Design review of the part built by this model. Coordinates are the model's own, in mm. Face numbers are marked on the shaded views. A direction names the side the tool comes from. Coordinates: 2 decimals unless noted, no trailing zeros. Order: outer loops, then holes, each group sorted by start corner. A loop starts at its lowest first (then second) coordinate and runs counter-clockwise, first axis right, second up. Notation, with made-up numbers: (-3.75, -17) -> (43.25, -17) arc R15 ccw to (43.25, 11) -> close; hole circle Ø11 at (18.5, -10.75). An arc over 180 degrees is marked (long way). Write item = value, one per line.
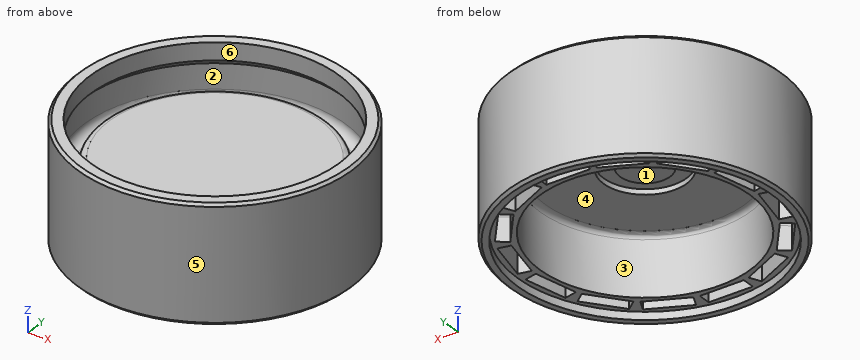
```python
from build123d import *

# Parameters (mm, degrees)
F0_R            = 26
F1_DEPTH        = 22
F2_W            = 8.4
F2_H            = 2.4
F3_DEPTH        = 10
F3_COPIES_COUNT = 14
F4_R            = 4
F5_R            = 20
F6_DEPTH        = 13
F7_R            = 7.9
F8_DEPTH        = 1
F9_R            = 4.75
F10_DEPTH       = 0.8
F11_R           = 23.6
F12_DEPTH       = 7
F13_R           = 24.8
F13_R_2         = 21.2
F14_DEPTH       = 4
F14_DEPTH_BACK  = 4
F15_R           = 1.79999
F16_R           = 1.2
F17_S5_R        = 23.6
F17_T6_DEPTH    = 37
F18_R           = 1
F19_SIZE        = 0.5
F20_R           = 24.3
F21_DEPTH       = 1.5


# Not quite as in the source:
# - a fillet or chamfer that OpenCascade refuses, or shapes differently, is made with other operations: its cross-section is extruded or revolved along the edge and cut away or added
# - a fillet or chamfer is up to 0.001 mm smaller than in the source, because OpenCascade refuses the exact size
# - a pattern or mirror of a feature is missing from the dataset's text; its kind, count and spacing are read off the source's solid


with BuildPart() as f1:
    # F0 (on Top) → F1 (new body)
    with BuildSketch(Plane.XY):
        Circle(F0_R)
    extrude(amount=F1_DEPTH)

    # F2 (on face) → F3 (cut)
    with BuildSketch(Plane(origin=(0, 0, 0), x_dir=(1, 0, 0), z_dir=(0, 0, -1))):
        with Locations((0, 22)):
            Rectangle(F2_W, F2_H)
    f3 = extrude(amount=-F3_DEPTH, mode=Mode.SUBTRACT)

    # F3_copies: F3 ×14 about axis
    f3_copies_axis = Axis((0, 0, 0), (0, 0, 1))
    for i in range(1, F3_COPIES_COUNT):
        add(f3.rotate(f3_copies_axis, i * 360 / F3_COPIES_COUNT), mode=Mode.SUBTRACT)

    # F4
    f4_edges = [f1.edges().sort_by_distance(p)[0] for p in [
        (4.2, -22, 10),
        (-4.2, -22, 10),
        (-19.81895, -10.433083, 10),
        (-14.581635, -17.000468, 10),
        (-13.329512, -17.999003, 10),
        (-5.761373, -21.643627, 10),
        (-22.383002, -0.800763, 10),
        (-20.513826, -8.990158, 10),
        (5.761373, -21.643627, 10),
        (13.329512, -17.999003, 10),
        (14.581635, -17.000468, 10),
        (19.81895, -10.433083, 10),
        (20.513826, -8.990158, 10),
        (22.383002, -0.800763, 10),
        (-20.513826, 8.990158, 10),
        (-22.383002, 0.800763, 10),
        (-14.581635, 17.000468, 10),
        (-19.81895, 10.433083, 10),
        (-5.761373, 21.643627, 10),
        (-13.329512, 17.999003, 10),
        (22.383002, 0.800763, 10),
        (20.513826, 8.990158, 10),
        (4.2, 22, 10),
        (-4.2, 22, 10),
        (13.329512, 17.999003, 10),
        (5.761373, 21.643627, 10),
        (19.81895, 10.433083, 10),
        (14.581635, 17.000468, 10),
    ]]
    fillet(f4_edges, radius=F4_R)

    # F5 (on face) → F6 (cut)
    with BuildSketch(Plane(origin=(0, 0, 0), x_dir=(1, 0, 0), z_dir=(0, 0, -1))):
        Circle(F5_R)
    extrude(amount=-F6_DEPTH, mode=Mode.SUBTRACT)

    # F7 (on face) → F8 (cut)
    with BuildSketch(Plane(origin=(0, 0, 13), x_dir=(1, 0, 0), z_dir=(0, 0, -1))):
        Circle(F7_R)
    extrude(amount=-F8_DEPTH, mode=Mode.SUBTRACT)

    # F9 (on face) → F10 (join)
    with BuildSketch(Plane(origin=(0, 0, 14), x_dir=(1, 0, 0), z_dir=(0, 0, -1))):
        Circle(F9_R)
    extrude(amount=F10_DEPTH)

    # F11 (on face) → F12 (cut)
    with BuildSketch(Plane.XY.offset(22)):
        Circle(F11_R)
    extrude(amount=-F12_DEPTH, mode=Mode.SUBTRACT)

    # F13 (on face) → F14 (cut, two sides)
    with BuildSketch(Plane.XY.offset(15)) as f14_sk:
        Circle(F13_R)
        Circle(F13_R_2, mode=Mode.SUBTRACT)
    extrude(amount=-F14_DEPTH, mode=Mode.SUBTRACT)
    extrude(f14_sk.sketch, amount=F14_DEPTH_BACK, mode=Mode.SUBTRACT)

    # F15 (radius 1.8 in the source; OpenCascade refuses exactly that, so slightly less here)
    f15_edges = [f1.edges().sort_by_distance(p)[0] for p in [
        (-24.8, 0, 11),
        (-21.2, 0, 11),
    ]]
    fillet(f15_edges, radius=F15_R)

    # F16
    f16_edges = [f1.edges().sort_by_distance(p)[0] for p in [
        (-21.2, 0, 15),
    ]]
    fillet(f16_edges, radius=F16_R)

    # F17: chamfer of 1.5 on 1 edges, made by hand


with BuildPart() as f17_tool2:
    # F17_s3 → F17_t4 (revolve)
    with BuildSketch(Plane.XZ):
        Polygon((24.8, 17.5), (23.3, 19), (24.8, 19), align=None)
    revolve(axis=Axis((0, 0, 19), (0, 0, 1)))

    # F17_s5 → F17_t6 (cut, symmetric)
    with BuildSketch(Plane.XY.offset(18.2)):
        Circle(F17_S5_R)
    extrude(amount=F17_T6_DEPTH, both=True, mode=Mode.SUBTRACT)


with BuildPart() as f1_1:
    add(f1.part)

    # F17_t1: union F17_tool2
    add(f17_tool2.part)

    # F18
    f18_edges = [f1_1.edges().sort_by_distance(p)[0] for p in [
        (-20, 0, 13),
    ]]
    fillet(f18_edges, radius=F18_R)

    # F19
    f19_edges = [f1_1.edges().sort_by_distance(p)[0] for p in [
        (-26, 0, 0),
        (-26, 0, 22),
    ]]
    chamfer(f19_edges, length=F19_SIZE)

    # F20 (on face) → F21 (cut)
    with BuildSketch(Plane(origin=(0, 0, 0), x_dir=(1, 0, 0), z_dir=(0, 0, -1))):
        Circle(F20_R)
    extrude(amount=-F21_DEPTH, mode=Mode.SUBTRACT)


solid = f1_1.part
```
(1) Insertion check: pin 1 (8 mm diameter, centred on x = -12.5, y = 11.5, fed in from +Z); pin 2 (1.4 mm diameter, centred on x = -16.5, y = -13.5, fed in from -Z); pin 3 (1 mm diameter, centred on x = -21, y = -5, fed in from -Z). Each pin has a flat end and moves straight along its axis. Give the tip position at first contact, or say it passes through.
Report:
pin_1 = 15
pin_2 = 1.5
pin_3 = 9.97
(2) We need section A-A (z = 20). Write out the cut boundary in (x, y).
Report:
outline = circle Ø52 at (0, 0); hole circle Ø47.2 at (0, 0)
(3) For the marked faces 4, 5 and 6, list the 3-axis set-ups (+Z, -Z, +X, -X, +Y, -Y) from which the entire face can be reached by the end or side of a thin tool; tool diameter is ignored.
Report:
face_4 = -Z
face_5 = +Z, -Z
face_6 = +Z
(4) The part is to be moulded in two halves that separate along Z. For the marked faces 1, 2 and 3, say which applies: released by +Z, released by -Z, zero draft, split by the parting line, or undercut.
Report:
face_1 = released by -Z
face_2 = undercut
face_3 = zero draft
(5) For L1, parallel to Y at x = 0, z = 13.65; L2, parallel to X at y = -4.5, z = 2; L3, parallel to Y at x = 0, z = 14.45, list the stretches that pass through material, from the lowest coordinate up.
Report:
L1 = -26 to -24.8, -21.2 to -7.9, -4.75 to 4.75, 7.9 to 21.2, 24.8 to 26
L2 = -25.61 to -22.77, -20.31 to -19.49, 19.49 to 20.31, 22.77 to 25.61
L3 = -26 to -24.8, -21.01 to 21.01, 24.8 to 26
